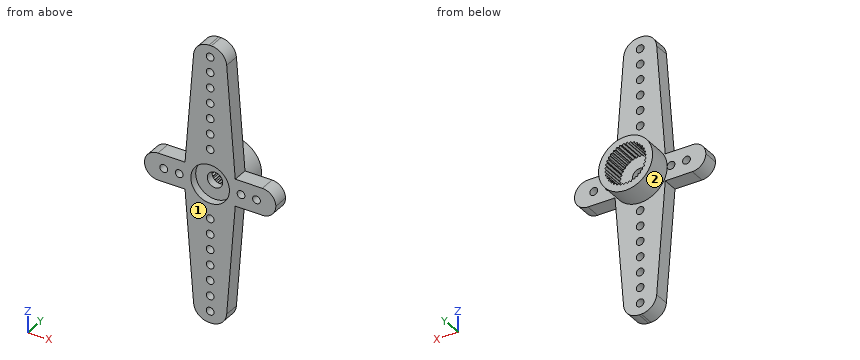
from build123d import *

# Parameters (mm, degrees)
BOSS_EXTRUDE1_DEPTH     = 2
FILLET1_R               = 2
FILLET2_R               = 1.75
SKETCH2_R               = 3.5
BOSS_EXTRUDE2_DEPTH     = 3
SKETCH3_R               = 2.5
CUT_EXTRUDE1_DEPTH      = 1
SKETCH4_R               = 1
CUT_EXTRUDE2_DEPTH      = 21.303940504
CUT_EXTRUDE3_START      = -3
SKETCH5_R               = 2.5
CUT_EXTRUDE3_DEPTH      = 3
CUT_EXTRUDE4_DEPTH      = 3
CIRPATTERN1_COUNT       = 36
SKETCH9_R               = 0.5
CUT_EXTRUDE5_DEPTH      = 21.524375752
LPATTERN1_COUNT         = 7
LPATTERN1_PITCH         = 2
MIRROR1_COPY_1_SKETCH_R = 0.5
MIRROR1_COPY_1_DEPTH    = 21.524375752
MIRROR1_COPY_2_SKETCH_R = 0.5
MIRROR1_COPY_2_DEPTH    = 21.524375752
MIRROR1_COPY_3_SKETCH_R = 0.5
MIRROR1_COPY_3_DEPTH    = 21.524375752
MIRROR1_COPY_4_SKETCH_R = 0.5
MIRROR1_COPY_4_DEPTH    = 21.524375752
MIRROR1_COPY_5_SKETCH_R = 0.5
MIRROR1_COPY_5_DEPTH    = 21.524375752
MIRROR1_COPY_6_SKETCH_R = 0.5
MIRROR1_COPY_6_DEPTH    = 21.524375752
SKETCH11_R              = 0.5
CUT_EXTRUDE6_DEPTH      = 21.524375752
LPATTERN2_COUNT         = 2
LPATTERN2_PITCH         = 2
MIRROR2_COPY_1_SKETCH_R = 0.5
MIRROR2_COPY_1_DEPTH    = 21.524375752


with BuildPart() as part:
    # Sketch1 → Boss-Extrude1 (new body)
    with BuildSketch(Plane(origin=(0, 0, 0), x_dir=(1, 0, 0), z_dir=(0, 1, 0))):
        Polygon((-8.5, 1.75), (-3.25, 1.75), (-2, 18), (2, 18), (3.25, 1.75), (8.5, 1.75), (8.5, -1.75), (3.25, -1.75), (2, -18), (-2, -18), (-3.25, -1.75), (-8.5, -1.75), align=None)
    extrude(amount=BOSS_EXTRUDE1_DEPTH)

    # Fillet1
    fillet1_edges = [part.edges().sort_by_distance(p)[0] for p in [
        (-2, 1, -18),
        (2, 1, -18),
        (2, 1, 18),
        (-2, 1, 18),
    ]]
    fillet(fillet1_edges, radius=FILLET1_R)

    # Fillet2
    fillet2_edges = [part.edges().sort_by_distance(p)[0] for p in [
        (-8.5, 1, -1.75),
        (-8.5, 1, 1.75),
        (8.5, 1, -1.75),
        (8.5, 1, 1.75),
    ]]
    fillet(fillet2_edges, radius=FILLET2_R - 0.0001)  # a hair under: the kernel refuses the full size

    # Sketch2 → Boss-Extrude2 (add)
    with BuildSketch(Plane(origin=(0, 2, 0), x_dir=(1, 0, 0), z_dir=(0, 1, 0))):
        with Locations(Location((0, 0, 0), (0, 0, 90))):
            Circle(SKETCH2_R)
    extrude(amount=BOSS_EXTRUDE2_DEPTH)

    # Sketch3 → Cut-Extrude1 (cut)
    with BuildSketch(Plane(origin=(0, 0, 0), x_dir=(-1, 0, 0), z_dir=(0, -1, 0))):
        with Locations(Location((0, 0, 0), (0, 0, 90))):
            Circle(SKETCH3_R)
    extrude(amount=-CUT_EXTRUDE1_DEPTH, mode=Mode.SUBTRACT)

    # Sketch4 → Cut-Extrude2 (cut, through all)
    with BuildSketch(Plane(origin=(0, 1, 0), x_dir=(-1, 0, 0), z_dir=(0, -1, 0))):
        with Locations(Location((0, 0, 0), (0, 0, 90))):
            Circle(SKETCH4_R)
    extrude(amount=-CUT_EXTRUDE2_DEPTH, mode=Mode.SUBTRACT)

    # Sketch5 → Cut-Extrude3 (cut)
    with BuildSketch(Plane(origin=(0, 5, 0), x_dir=(1, 0, 0), z_dir=(0, 1, 0)).offset(CUT_EXTRUDE3_START)):
        with Locations(Location((0, 0, 0), (0, 0, 90))):
            Circle(SKETCH5_R)
    extrude(amount=CUT_EXTRUDE3_DEPTH, mode=Mode.SUBTRACT)

    # Sketch6 → Cut-Extrude4 (cut)
    with BuildSketch(Plane(origin=(0, 5, 0), x_dir=(1, 0, 0), z_dir=(0, 1, 0))):
        Polygon((-2.5, 0), (-2.691676801, 0.211839558), (-2.469220851, 0.391086163), align=None)
    cut_extrude4 = extrude(amount=-CUT_EXTRUDE4_DEPTH, mode=Mode.SUBTRACT)

    # CirPattern1: Cut-Extrude4 ×36 about axis
    cirpattern1_axis = Axis((0, 0, 0), (0, 1, 0))
    for i in range(1, CIRPATTERN1_COUNT):
        add(cut_extrude4.rotate(cirpattern1_axis, i * 360 / CIRPATTERN1_COUNT), mode=Mode.SUBTRACT)

    # Sketch9 → Cut-Extrude5 (cut, through all)
    with BuildSketch(Plane(origin=(0, 0, 0), x_dir=(-1, 0, 0), z_dir=(0, -1, 0))):
        with Locations(Location((0, 16.5, 0), (0, 0, 90))):
            Circle(SKETCH9_R)
    cut_extrude5 = extrude(amount=-CUT_EXTRUDE5_DEPTH, mode=Mode.SUBTRACT)

    # LPattern1: Cut-Extrude5 ×7
    with Locations(*[(0, 0, i * LPATTERN1_PITCH) for i in range(1, LPATTERN1_COUNT)]):
        add(cut_extrude5, mode=Mode.SUBTRACT)

    # Mirror1: Cut-Extrude5 across plane
    add(cut_extrude5.mirror(Plane.XY), mode=Mode.SUBTRACT)

    # Mirror1 copy 1 sketch → Mirror1 copy 1 (cut, through all)
    with BuildSketch(Plane(origin=(0, 0, -2), x_dir=(-1, 0, 0), z_dir=(0, -1, 0))):
        with Locations((0, -16.5)):
            Circle(MIRROR1_COPY_1_SKETCH_R)
    extrude(amount=-MIRROR1_COPY_1_DEPTH, mode=Mode.SUBTRACT)

    # Mirror1 copy 2 sketch → Mirror1 copy 2 (cut, through all)
    with BuildSketch(Plane(origin=(0, 0, -4), x_dir=(-1, 0, 0), z_dir=(0, -1, 0))):
        with Locations((0, -16.5)):
            Circle(MIRROR1_COPY_2_SKETCH_R)
    extrude(amount=-MIRROR1_COPY_2_DEPTH, mode=Mode.SUBTRACT)

    # Mirror1 copy 3 sketch → Mirror1 copy 3 (cut, through all)
    with BuildSketch(Plane(origin=(0, 0, -6), x_dir=(-1, 0, 0), z_dir=(0, -1, 0))):
        with Locations((0, -16.5)):
            Circle(MIRROR1_COPY_3_SKETCH_R)
    extrude(amount=-MIRROR1_COPY_3_DEPTH, mode=Mode.SUBTRACT)

    # Mirror1 copy 4 sketch → Mirror1 copy 4 (cut, through all)
    with BuildSketch(Plane(origin=(0, 0, -8), x_dir=(-1, 0, 0), z_dir=(0, -1, 0))):
        with Locations((0, -16.5)):
            Circle(MIRROR1_COPY_4_SKETCH_R)
    extrude(amount=-MIRROR1_COPY_4_DEPTH, mode=Mode.SUBTRACT)

    # Mirror1 copy 5 sketch → Mirror1 copy 5 (cut, through all)
    with BuildSketch(Plane(origin=(0, 0, -10), x_dir=(-1, 0, 0), z_dir=(0, -1, 0))):
        with Locations((0, -16.5)):
            Circle(MIRROR1_COPY_5_SKETCH_R)
    extrude(amount=-MIRROR1_COPY_5_DEPTH, mode=Mode.SUBTRACT)

    # Mirror1 copy 6 sketch → Mirror1 copy 6 (cut, through all)
    with BuildSketch(Plane(origin=(0, 0, -12), x_dir=(-1, 0, 0), z_dir=(0, -1, 0))):
        with Locations((0, -16.5)):
            Circle(MIRROR1_COPY_6_SKETCH_R)
    extrude(amount=-MIRROR1_COPY_6_DEPTH, mode=Mode.SUBTRACT)

    # Sketch11 → Cut-Extrude6 (cut, through all)
    with BuildSketch(Plane(origin=(0, 0, 0), x_dir=(-1, 0, 0), z_dir=(0, -1, 0))):
        with Locations(Location((-6, 0, 0), (0, 0, 90))):
            Circle(SKETCH11_R)
    cut_extrude6 = extrude(amount=-CUT_EXTRUDE6_DEPTH, mode=Mode.SUBTRACT)

    # LPattern2: Cut-Extrude6 ×2
    with Locations(*[(-i * LPATTERN2_PITCH, 0, 0) for i in range(1, LPATTERN2_COUNT)]):
        add(cut_extrude6, mode=Mode.SUBTRACT)

    # Mirror2: Cut-Extrude6 across plane
    add(cut_extrude6.mirror(Plane(origin=(0, 0, 0), x_dir=(0, 0, 1), z_dir=(1, 0, 0))), mode=Mode.SUBTRACT)

    # Mirror2 copy 1 sketch → Mirror2 copy 1 (cut, through all)
    with BuildSketch(Plane(origin=(2, 0, 0), x_dir=(1, 0, 0), z_dir=(0, -1, 0))):
        with Locations((-6, 0)):
            Circle(MIRROR2_COPY_1_SKETCH_R)
    extrude(amount=-MIRROR2_COPY_1_DEPTH, mode=Mode.SUBTRACT)


solid = part.part
Build history of the part. All positions in model axes, mm. Face numbers are marked on the shaded views. A direction names the side the tool comes from. Give positions to 0.01 mm unless a question says otherwise; leave off trailing zeros. Order: outer loops, then holes, each group sorted by start corner. A loop starts at its lowest first (then second) coordinate and runs counter-clockwise, first axis right, second up. Notation, with made-up numbers: M -3,40.25 L 22,40.25 A12 ccw 22,52.25 Z; hole C 25.25,5.25 d9. An arc over 180 degrees is marked long. Use one line per item in the form item = value.
Q1. Which spindle directions (+Z, -Z, +X, -X, +Y, -Y) get a long thin tool onto all of the face, cutting with end or side? Do the marked faces 1 and 2. Say none if no direction does.
Conclusion:
face_1 = +Z, -Z, +X, -X, -Y
face_2 = +Y
Q2. Slice it at C-C, the plane y = 1.6. State how many separate pieces and enclosed holes the cut face has, and give its area (3 significant figures).
Conclusion:
separate_pieces = 1
enclosed_holes = 19
area = 207 mm2
Q3. Slice it at A-A, the plane x = 4. Write the cut outline in (y, z), and give its area (3 significant figures).
Conclusion:
outline = M 0,-1.75 L 2,-1.75 L 2,-0.5 L 0,-0.5 Z; M 0,0.5 L 2,0.5 L 2,1.75 L 0,1.75 Z
area = 5.00 mm2
Q4. Pin check, flat tips, straight feed: P1, Ø0.6, axis at x = 4.5, y = 1.5, coming from the -Z side; P2, Ø1.5, axis at x = 0.5, z = -11.5, coming from the +Y side; P3, Ø1.5, axis at x = 1, z = 1, coming from the -Y side. Stop position of each tip, or through.
Conclusion:
P1 = -1.75
P2 = 2
P3 = 1
Q5. Slice it at B-B, the plane z = -12.5. Write the cut outline in (x, y), and give its area (3 significant figures).
Conclusion:
outline = M -2.42,0 L -0.5,0 L -0.5,2 L -2.42,2 Z; M 0.5,0 L 2.42,0 L 2.42,2 L 0.5,2 Z
area = 7.69 mm2
Q6. Slice it at D-D, the plane z = 7.5. Write the cut outline in (x, y).
Conclusion:
outline = M -2.81,0 L 2.81,0 L 2.81,2 L -2.81,2 Z
Q7. Wall check: probe 1 along Z at (x, y) = (-6, 0.5); probe 2 along Y at (x, z) = (-1.25, 8.5); probe 3 along X at (y, z) = (0.4, 8.5). Give the ranges that are in metal, low to high.
Conclusion:
probe_1 = -1.75 to -0.5, 0.5 to 1.75
probe_2 = 0 to 2
probe_3 = -2.73 to -0.5, 0.5 to 2.73
